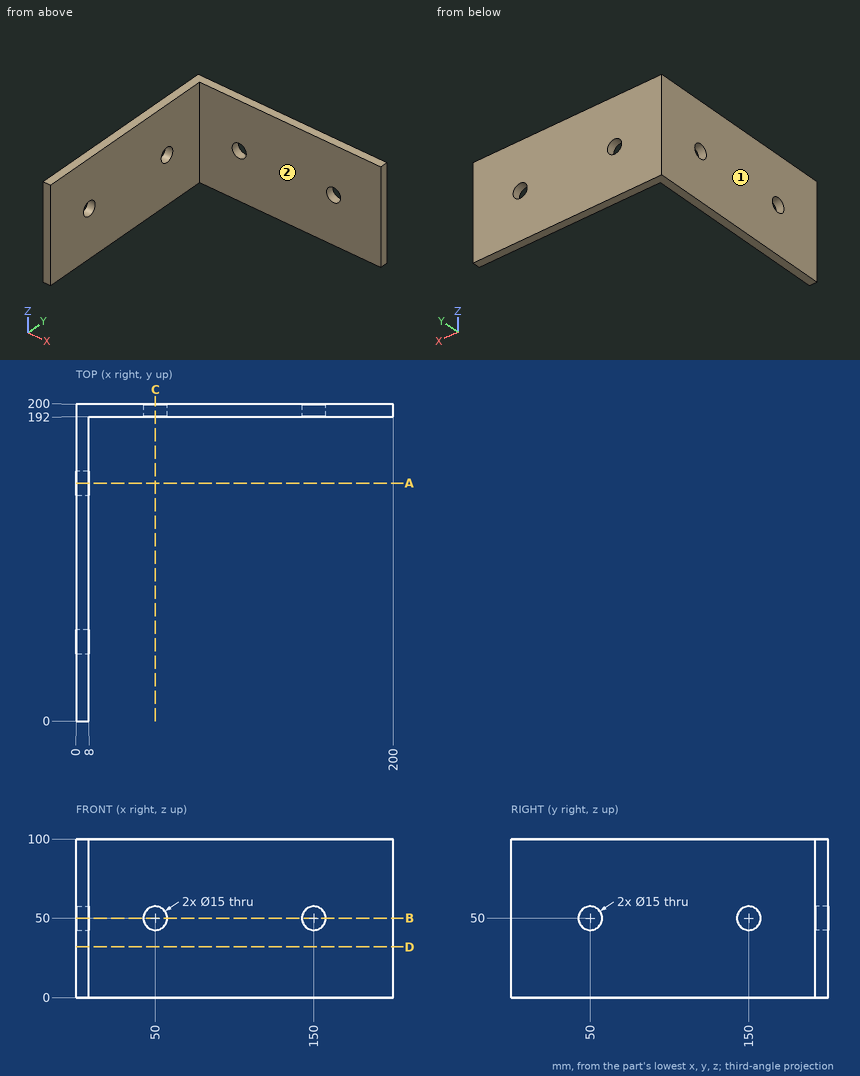
Job drawing, mm, ordinate dimensions from the low corner. One solid piece. A direction names the side the tool comes from. Coordinates: 2 decimals unless noted, no trailing zeros. Order: outer loops, then holes, each group sorted by start corner. A loop starts at its lowest first (then second) coordinate and runs counter-clockwise, first axis right, second up. Notation, with made-up numbers: M 45,44 L 63,44 A17 ccw 63,49 Z; hole C -7.5,-9 d5. An arc over 180 degrees is marked long. Answer as CSV lines item,"result".
(1) Band-saw the part on A-A, the plane y = 150. List the corners of the cut face in (x, z), then the cut area to 3 significant figures.
Geometry says:
outline,"M 0,0 L 8,0 L 8,42.5 L 0,42.5 Z; M 0,57.5 L 8,57.5 L 8,100 L 0,100 Z"
area,"680 mm2"
(2) Flat gauge pins, fed straight in: pin 1 (17 mm diameter, centred on y = 50, z = 50, fed in from +X); pin 2 (9 mm diameter, centred on y = 150, z = 50, fed in from -X); pin 3 (6 mm diameter, centred on x = 20.5, z = 61, fed in from -Y). Where does each tip first touch, or does it go through?
Geometry says:
pin 1,"stops at x = 8"
pin 2,"passes through"
pin 3,"stops at y = 192"
(3) Band-saw the part on B-B, the plane z = 50. List the corners of the cut face in (x, y), then the cut area to 3 significant figures.
Geometry says:
outline,"M 0,0 L 8,0 L 8,42.5 L 0,42.5 Z; M 0,57.5 L 8,57.5 L 8,142.5 L 0,142.5 Z; M 0,157.5 L 8,157.5 L 8,192 L 42.5,192 L 42.5,200 L 0,200 Z; M 57.5,192 L 142.5,192 L 142.5,200 L 57.5,200 Z; M 157.5,192 L 200,192 L 200,200 L 157.5,200 Z"
area,"2,660 mm2"
(4) Band-saw the part on D-D, the plane z = 32. List the corners of the cut face in (x, y).
Geometry says:
outline,"M 0,0 L 8,0 L 8,192 L 200,192 L 200,200 L 0,200 Z"
(5) Band-saw the part on C-C, the plane x = 50. List the corners of the cut face in (y, z), then the cut area to 3 significant figures.
Geometry says:
outline,"M 192,0 L 200,0 L 200,42.5 L 192,42.5 Z; M 192,57.5 L 200,57.5 L 200,100 L 192,100 Z"
area,"680 mm2"
(6) 3-axis set-ups, long thin cutter, end or side, ignore diameter. For the marked faces 1 and 2: which of +Z, -Z, +X, -X, +Y, -Y reach the whole face in a straight line?
Geometry says:
face 1,"+Z, -Z, -X, +Y, -Y"
face 2,"+Z, -Z, +X, -Y"
(7) Wall check: line 1 along Z through (x, y) = (50, 196); line 2 along Y through (x, z) = (53, 65); line 3 along X through (y, z) = (121, 12). Give the ranges that are in metal, low to high.
Geometry says:
line 1,"z = 0 to 42.5, 57.5 to 100"
line 2,"y = 192 to 200"
line 3,"x = 0 to 8"
